Part model, mm, in its own coordinate system. Round coordinates to 2 decimals unless told otherwise and drop trailing zeros. One line per question, with ' | ' between items. Start each with the question number.
1) Drop flat-ended pins along their axis: pin 1 Ø0.6 at (y, z) = (-2, 3) entering from -X; pin 2 Ø1 at (x, z) = (25, 2.5) entering from -Y; pin 3 Ø0.6 at (x, z) = (-1.5, 4) entering from +Y. Give the stop position or say it passes through.
2) Wall check: probe 1 along Y at (x, z) = (1.5, 7); probe 2 along Y at (x, z) = (17, 2.25); probe 3 along X at (y, z) = (1, 2.5). Give the ranges that are in metal, low to high. Write a range as [from, to].
3) Saw through at A-A (z = 3.5). Give the number of separate pieces and of enclosed holes in the cut face, plus the area to 3 significant figures.
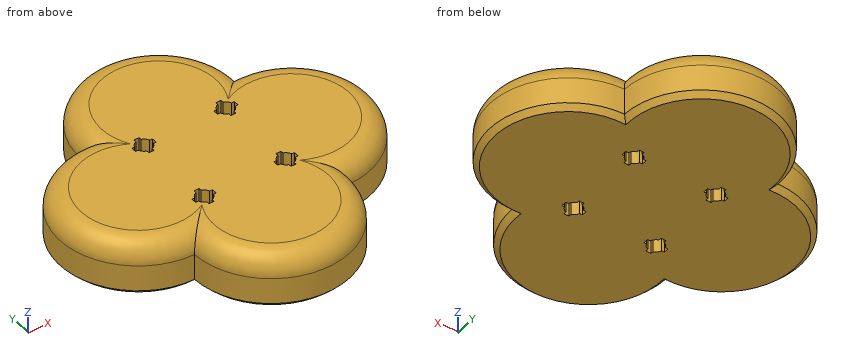
```python
from build123d import *

# Parameters (mm, degrees)
BOSS_EXTRUDE1_DEPTH = 10
FILLET1_R           = 4
CHAMFER1_SIZE       = 1


with BuildPart() as part:
    # Sketch1 → Boss-Extrude1 (new body)
    with BuildSketch(Plane.XY):
        with BuildLine():
            ThreePointArc((-7, 7), (8, 22), (23, 7))
            ThreePointArc((23, 7), (38, -8), (23, -23))
            ThreePointArc((23, -23), (8, -38), (-7, -23))
            ThreePointArc((-7, -23), (-22, -8), (-7, 7))
        make_face()
        with BuildLine():
            Line((-0.5, -2), (0.5, -2))
            Line((0.5, -2), (0.5, -1.467140075))
            ThreePointArc((0.5, -1.467140075), (1.096015511, -1.096015511), (1.467140075, -0.5))
            Line((1.467140075, -0.5), (2, -0.5))
            Line((2, -0.5), (2, 0.5))
            Line((2, 0.5), (1.467140075, 0.5))
            ThreePointArc((1.467140075, 0.5), (1.096015511, 1.096015511), (0.5, 1.467140075))
            Line((0.5, 1.467140075), (0.5, 2))
            Line((0.5, 2), (-0.5, 2))
            Line((-0.5, 2), (-0.5, 1.467140075))
            ThreePointArc((-0.5, 1.467140075), (-1.096015511, 1.096015511), (-1.467140075, 0.5))
            Line((-1.467140075, 0.5), (-2, 0.5))
            Line((-2, 0.5), (-2, -0.5))
            Line((-2, -0.5), (-1.467140075, -0.5))
            ThreePointArc((-1.467140075, -0.5), (-1.096015511, -1.096015511), (-0.5, -1.467140075))
            Line((-0.5, -1.467140075), (-0.5, -2))
        make_face(mode=Mode.SUBTRACT)
        with BuildLine():
            Line((18, -0.5), (18, 0.5))
            Line((18, 0.5), (17.467140075, 0.5))
            ThreePointArc((17.467140075, 0.5), (17.096015511, 1.096015511), (16.5, 1.467140075))
            Line((16.5, 1.467140075), (16.5, 2))
            Line((16.5, 2), (15.5, 2))
            Line((15.5, 2), (15.5, 1.467140075))
            ThreePointArc((15.5, 1.467140075), (14.903984489, 1.096015511), (14.532859925, 0.5))
            Line((14.532859925, 0.5), (14, 0.5))
            Line((14, 0.5), (14, -0.5))
            Line((14, -0.5), (14.532859925, -0.5))
            ThreePointArc((14.532859925, -0.5), (14.903984489, -1.096015511), (15.5, -1.467140075))
            Line((15.5, -1.467140075), (15.5, -2))
            Line((15.5, -2), (16.5, -2))
            Line((16.5, -2), (16.5, -1.467140075))
            ThreePointArc((16.5, -1.467140075), (17.096015511, -1.096015511), (17.467140075, -0.5))
            Line((17.467140075, -0.5), (18, -0.5))
        make_face(mode=Mode.SUBTRACT)
        with BuildLine():
            Line((18, -15.5), (17.467140075, -15.5))
            ThreePointArc((17.467140075, -15.5), (17.096015511, -14.903984489), (16.5, -14.532859925))
            Line((16.5, -14.532859925), (16.5, -14))
            Line((16.5, -14), (15.5, -14))
            Line((15.5, -14), (15.5, -14.532859925))
            ThreePointArc((15.5, -14.532859925), (14.903984489, -14.903984489), (14.532859925, -15.5))
            Line((14.532859925, -15.5), (14, -15.5))
            Line((14, -15.5), (14, -16.5))
            Line((14, -16.5), (14.532859925, -16.5))
            ThreePointArc((14.532859925, -16.5), (14.903984489, -17.096015511), (15.5, -17.467140075))
            Line((15.5, -17.467140075), (15.5, -18))
            Line((15.5, -18), (16.5, -18))
            Line((16.5, -18), (16.5, -17.467140075))
            ThreePointArc((16.5, -17.467140075), (17.096015511, -17.096015511), (17.467140075, -16.5))
            Line((17.467140075, -16.5), (18, -16.5))
            Line((18, -16.5), (18, -15.5))
        make_face(mode=Mode.SUBTRACT)
        with BuildLine():
            Line((-2, -15.5), (-2, -16.5))
            Line((-2, -16.5), (-1.467140075, -16.5))
            ThreePointArc((-1.467140075, -16.5), (-1.096015511, -17.096015511), (-0.5, -17.467140075))
            Line((-0.5, -17.467140075), (-0.5, -18))
            Line((-0.5, -18), (0.5, -18))
            Line((0.5, -18), (0.5, -17.467140075))
            ThreePointArc((0.5, -17.467140075), (1.096015511, -17.096015511), (1.467140075, -16.5))
            Line((1.467140075, -16.5), (2, -16.5))
            Line((2, -16.5), (2, -15.5))
            Line((2, -15.5), (1.467140075, -15.5))
            ThreePointArc((1.467140075, -15.5), (1.096015511, -14.903984489), (0.5, -14.532859925))
            Line((0.5, -14.532859925), (0.5, -14))
            Line((0.5, -14), (-0.5, -14))
            Line((-0.5, -14), (-0.5, -14.532859925))
            ThreePointArc((-0.5, -14.532859925), (-1.096015511, -14.903984489), (-1.467140075, -15.5))
            Line((-1.467140075, -15.5), (-2, -15.5))
        make_face(mode=Mode.SUBTRACT)
    extrude(amount=BOSS_EXTRUDE1_DEPTH)

    # Fillet1
    fillet1_edges = [part.edges().sort_by_distance(p)[0] for p in [
        (-22, -8, 10),
        (8, -38, 10),
        (38, -8, 10),
        (8, 22, 10),
    ]]
    fillet(fillet1_edges, radius=FILLET1_R)

    # Chamfer1
    chamfer1_edges = [part.edges().sort_by_distance(p)[0] for p in [
        (38, -8, 0),
        (8, -38, 0),
        (-22, -8, 0),
        (8, 22, 0),
    ]]
    chamfer(chamfer1_edges, length=CHAMFER1_SIZE)


solid = part.part
```
Answer key:
1) pin 1: stops at x = -20.87 | pin 2: stops at y = -22.92 | pin 3: stops at y = 18.85
2) probe 1: y = [-36.38, -16.5], [-15.5, -0.5], [0.5, 20.38] | probe 2: y = [-35, -17.18], [-14.82, -1.18], [1.18, 19] | probe 3: x = [-19, -1.18], [1.18, 14.82], [17.18, 35]
3) separate pieces: 1 | enclosed holes: 4 | area: 2,280 mm2
